```python
from build123d import *

# Parameters (mm, degrees)
SWEEP_1_PROFILE_R   = 25
SKETCH_9_R          = 40
EXTRUDE_2_DEPTH     = 20
FILLET_1_R          = 5
SKETCH_11_W         = 60
SKETCH_11_H         = 15
EXTRUDE_3_DEPTH     = 200
CUT_EXTRUDE_1_DEPTH = 326.969707196
SCALE_1_SCALE       = 0.05


with BuildPart() as part:
    # 扫描1: sweep along a path in 草图1
    with BuildLine(Plane.XY) as sweep_1_path:
        Line((0, 0), (0, 100))
    # 扫描1 profile (on start of the path) → 扫描1 (sweep)
    with BuildSketch(Plane.ZX):
        Circle(SWEEP_1_PROFILE_R)
    sweep(path=sweep_1_path.line)

    # 草图9 → 凸台-拉伸2 (add)
    with BuildSketch(Plane(origin=(0, 100, 0), x_dir=(1, 0, 0), z_dir=(0, 1, 0))):
        with Locations(Location((0, 0, 0), (0, 0, 270))):
            Circle(SKETCH_9_R)
    extrude(amount=EXTRUDE_2_DEPTH)

    # 圆角1
    fillet_1_edges = [part.edges().sort_by_distance(p)[0] for p in [
        (0, 0, -25),
        (0, 100, -40),
        (0, 120, -40),
    ]]
    fillet(fillet_1_edges, radius=FILLET_1_R)

    # 草图11 → 凸台-拉伸3 (add)
    with BuildSketch(Plane(origin=(0, 120, 0), x_dir=(1, 0, 0), z_dir=(0, 1, 0))):
        Rectangle(SKETCH_11_W, SKETCH_11_H)
    extrude(amount=EXTRUDE_3_DEPTH)

    # 草图12 → 切除-拉伸1 (cut, through all)
    with BuildSketch(Plane.XY.offset(7.5)):
        with BuildLine():
            Line((-30, 224.261621757), (-30, 320))
            Line((-30, 320), (30, 320))
            ThreePointArc((30, 320), (-13.760497544, 280.754623688), (-30, 224.261621757))
        make_face()
    extrude(amount=-CUT_EXTRUDE_1_DEPTH, mode=Mode.SUBTRACT)


with BuildPart() as part_1:
    # 缩放比例1: scaled about (0.729315594, 117.844803008, 0)
    add(part.part.scale(SCALE_1_SCALE).moved(Location((0.692849814, 111.952562858, 0))))


solid = part_1.part
```
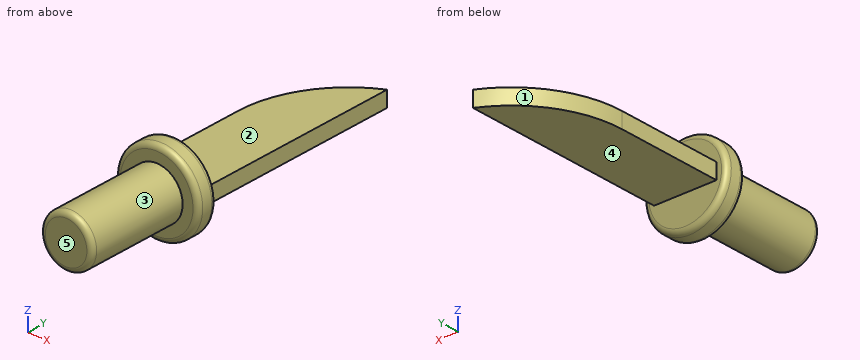
Input: part model. Units: mm. Frame: model coordinates. Face numbers are marked on the shaded views. A direction names the side the tool comes from. Give positions to 0.01 mm unless a question says otherwise; leave off trailing zeros. Order: outer loops, then holes, each group sorted by start corner. A loop starts at its lowest first (then second) coordinate and runs counter-clockwise, first axis right, second up.
1. Cut plane C-C (y = 115.5). Return loops of the section in (x, z).
Computed:
outline: circle Ø2.5 at (0.69, 0)
2. Set-up query: the marked faces 1, 2, 3, 4 and 5. Return all of +Z, -Z, +X, -X, +Y, -Y with unobstructed straight access to the full face (end or side cutting, diameter ignored); none if empty.
Computed:
face 1: +Z, -Z, -X, +Y
face 2: +Z, +X, -X, +Y
face 3: -Y
face 4: -Z, +X, -X, +Y
face 5: +Z, -Z, +X, -X, -Y
3. Line query: probe 1 along Z at (x, y) = (1.7, 119) (3 decimals); probe 2 along Y at (x, z) = (0.15, 1.6); probe 3 along Y at (x, z) = (0.25, -0.8). Output: solid intervals per line, ascending.
Computed:
probe 1: z = -0.375 to 0.375
probe 2: y = 116.95 to 117.95
probe 3: y = 111.95 to 117.95
4. Pin query (flat end, axial travel): pin 1 Ø1 at (y, z) = (121, -1) entering from +X; pin 2 Ø0.8 at (y, z) = (120, 0) entering from -X; pin 3 Ø0.9 at (x, y) = (1, 120.5) entering from -Z (3 decimals); pin 4 Ø1.5 at (x, y) = (1, 124.5) entering from +Z (3 decimals). Return the tip coordinate at first contact, or that it passes through.
Computed:
pin 1: passes through
pin 2: stops at x = -0.81
pin 3: stops at z = -0.375
pin 4: stops at z = 0.375
5. Cut plane B-B (y = 127.25). Return loops of the section in (x, z) (3 decimals).
Computed:
outline: (1.104, -0.375) - (2.193, -0.375) - (2.193, 0.375) - (1.104, 0.375) - close
6. Cut plane A-A (z = 0). Return loops of the section in (x, y), and give its area (3 significant figures).
Computed:
outline: (-1.31, 117.2) arc R0.25 ccw to (-1.06, 116.95) - (-0.56, 116.95) - (-0.56, 112.2) arc R0.25 ccw to (-0.31, 111.95) - (1.69, 111.95) arc R0.25 ccw to (1.94, 112.2) - (1.94, 116.95) - (2.44, 116.95) arc R0.25 ccw to (2.69, 117.2) - (2.69, 117.7) arc R0.25 ccw to (2.44, 117.95) - (2.19, 117.95) - (2.19, 127.95) arc R5.32 ccw to (-0.81, 123.17) - (-0.81, 117.95) - (-1.06, 117.95) arc R0.25 ccw to (-1.31, 117.7) - close
area: 42.3 mm2
